```python
from build123d import *

# Parameters (mm, degrees)
BOSS_EXTRUDE2_DEPTH                                = 76.2
CSK_FOR_10_FLAT_HEAD_MACHINE_SCREW_100_D           = 5.1054
CSK_FOR_10_FLAT_HEAD_MACHINE_SCREW_100_CSINK_D     = 9.779
CSK_FOR_10_FLAT_HEAD_MACHINE_SCREW_100_CSINK_ANGLE = 100


with BuildPart() as part:
    # Sketch1 → Boss-Extrude2 (new body)
    with BuildSketch(Plane(origin=(0, 0, 0), x_dir=(0, 0, -1), z_dir=(1, 0, 0))):
        with BuildLine():
            Line((0, 0), (0, 63.5))
            Line((0, 63.5), (3.81, 63.5))
            ThreePointArc((3.81, 63.5), (5.606051224, 62.756051224), (6.35, 60.96))
            Line((6.35, 60.96), (6.35, 8.89))
            ThreePointArc((6.35, 8.89), (7.093948776, 7.093948776), (8.89, 6.35))
            Line((8.89, 6.35), (60.96, 6.35))
            ThreePointArc((60.96, 6.35), (62.756051224, 5.606051224), (63.5, 3.81))
            Line((63.5, 3.81), (63.5, 0))
            Line((63.5, 0), (0, 0))
        make_face()
    extrude(amount=BOSS_EXTRUDE2_DEPTH)

    # CSK for #10 Flat Head Machine Screw (100)1 (through all)
    with Locations(Plane.XZ):
        with Locations((24.841747853, -48.183252147), (51.358252147, -48.183252147), (51.358252147, -21.666747853), (24.841747853, -21.666747853)):
            CounterSinkHole(CSK_FOR_10_FLAT_HEAD_MACHINE_SCREW_100_D / 2, CSK_FOR_10_FLAT_HEAD_MACHINE_SCREW_100_CSINK_D / 2, counter_sink_angle=CSK_FOR_10_FLAT_HEAD_MACHINE_SCREW_100_CSINK_ANGLE)


solid = part.part
```
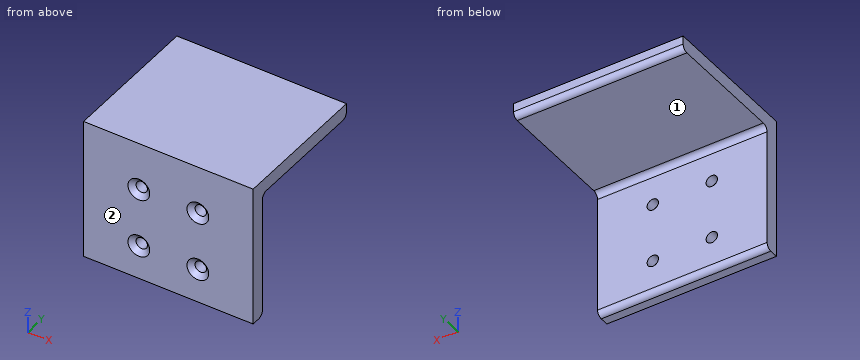
Can you work these out from the model? Positions are in its coordinate system, mm. Face numbers are marked on the shaded views. A direction names the side the tool comes from. Coordinates: 2 decimals unless noted, no trailing zeros. Write each loop counter-clockwise with the first axis right and the second up, starting at its lowest first coordinate (ties: lowest second). Pieces come first, ordered by that corner, then holes. Notation, with made-up numbers: (89, 58.5) - (110, 58.5) arc R21 ccw to (110, 91.5) - close; hole circle Ø7 at (18, -14.5). An arc over 180 degrees is marked (long way). Return JSON: item names as keys, results as strings.
Q1. If we section it at A-A (x = 61): Please give me the cut outline in (y, z).
Computed values:
{"outline": "(0, -63.5) - (3.81, -63.5) arc R2.54 ccw to (6.35, -60.96) - (6.35, -8.89) arc R2.54 cw to (8.89, -6.35) - (60.96, -6.35) arc R2.54 ccw to (63.5, -3.81) - (63.5, 0) - (0, 0) - close"}
Q2. If we section it at C-C (y = 25.5): Please give me the cut outline in (x, z).
Computed values:
{"outline": "(0, -6.35) - (76.2, -6.35) - (76.2, 0) - (0, 0) - close"}
Q3. If we section it at D-D (z = -55.5): Please give me the cut outline in (x, y), then the cut area to 3 significant figures.
Computed values:
{"outline": "(0, 0) - (76.2, 0) - (76.2, 6.35) - (0, 6.35) - close", "area": "484 mm2"}
Q4. If we section it at B-B (z = -47): Count the separate pieces of the cut face and the enclosed holes in it, then the cut area to 3 significant figures.
Computed values:
{"separate pieces": "3", "enclosed holes": "0", "area": "417 mm2"}
Q5. I'm going to push flat-ended pins straight in: pin 1 Ø15.5 at (x, z) = (43, -23.5) entering from +Y; pin 2 Ø4 at (x, y) = (54, 37.5) entering from -Z; pin 3 Ø4.5 at (x, z) = (24.84, -21.67) entering from -Y; pin 4 Ø8 at (x, z) = (51.36, -48.18) entering from -Y. Where does each tip first touch, or does it pass through?
Computed values:
{"pin 1": "stops at y = 6.35", "pin 2": "stops at z = -6.35", "pin 3": "passes through", "pin 4": "stops at y = 0.74"}
Q6. Please list where these lines run through material, in increasing order: L1, parallel to Y at x = 22, z = -16; L2, parallel to Z at x = 71.5, y = 13. Write a range as from..to.
Computed values:
{"L1": "y = 0..6.35", "L2": "z = -6.35..0"}
Q7. On a 3-axis mill with a long thin cutter (end or side, diameter ignored), from which of +Z, -Z, +X, -X, +Y, -Y can I reach the whole of each face in a straight line? I mean the marked faces 1 and 2. Say none if no direction works.
Computed values:
{"face 1": "-Z, +X, -X, +Y", "face 2": "+Z, -Z, +X, -X, -Y"}
